Check sheet for the drawn part. Datum: minimum x, y, z corner. Units: mm. A direction names the side the tool comes from. Give positions to 0.01 mm unless a question says otherwise; leave off trailing zeros. Loops run counter-clockwise (first coordinate to the right, second up) from the corner with the lowest first, then second, coordinate; pieces in that order, holes last. Notation, with made-up numbers: (62, 79) -> (118, 79) arc R36 cw to (118, 113) -> close; hole circle Ø11 at (6, 26). An arc over 180 degrees is marked (long way). One line per question, with ' | ' between items.
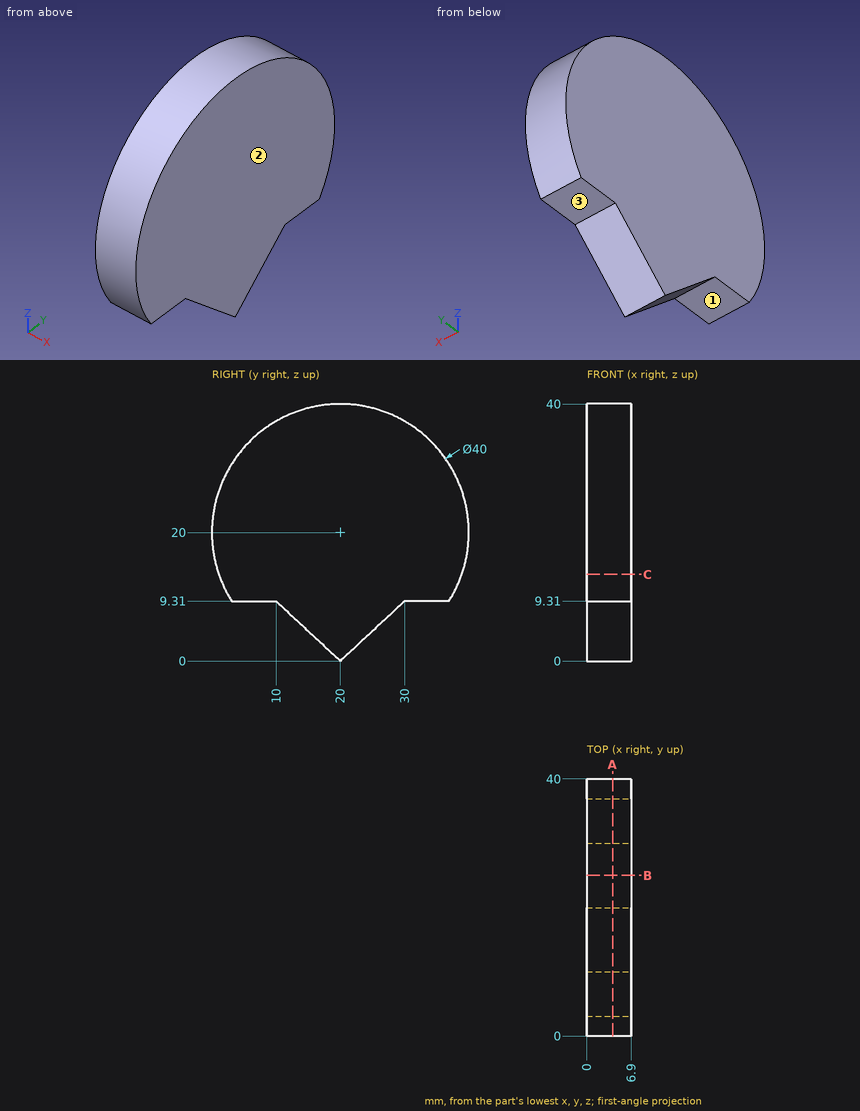
Item 1: Set-up check for the marked faces 1, 2 and 3: record each of +Z, -Z, +X, -X, +Y, -Y from which the full face is reachable in a straight line by a thin tool's end or side.
Result:
face 1: -Z, +X, -X, -Y | face 2: +Z, -Z, +X, +Y, -Y | face 3: -Z, +X, -X, +Y
Item 2: Depth check by flat-ended pin: pin 1 Ø1.5 at (x, y) = (3, 7.5) entering from -Z. Enter the tip coordinate at first touch or a pass-through.
Result:
pin 1: z = 9.31
Item 3: Scan lines: probe 1 along Z at (x, y) = (1.25, 27.5); probe 2 along Y at (x, z) = (4.75, 18.5); probe 3 along Z at (x, y) = (5.25, 27) (3 decimals). Record each from-to range of solid material in increasing order.
Result:
probe 1: 6.98 to 38.54 | probe 2: 0.06 to 39.94 | probe 3: 6.517 to 38.735
Item 4: Sectioned sample at A-A (x = 4). Record the cut outline in (y, z), plus the area to 3 significant figures.
Result:
outline: (3.1, 9.31) -> (10, 9.31) -> (20, 0) -> (30, 9.31) -> (36.9, 9.31) arc R20 ccw (long way) to start | area: 1,130 mm2
Item 5: Sectioned sample at C-C (z = 13.5). Record the cut outline in (x, y), plus the area to 3 significant figures.
Result:
outline: (0, 1.09) -> (6.9, 1.09) -> (6.9, 38.91) -> (0, 38.91) -> close | area: 261 mm2
Item 6: Sectioned sample at B-B (y = 25). Record the cut outline in (x, z) (3 decimals), plus the area to 3 significant figures.
Result:
outline: (0, 4.655) -> (6.9, 4.655) -> (6.9, 39.365) -> (0, 39.365) -> close | area: 239 mm2
